Input: part model. Units: mm. Frame: model coordinates. Face numbers are marked on the shaded views. A direction names the side the tool comes from. Give positions to 0.01 mm unless a question says otherwise; leave off trailing zeros. Write each loop counter-clockwise with the first axis right and the second up, starting at its lowest first coordinate (ties: lowest second). Pieces come first, ordered by that corner, then holes. Notation, with made-up numbers: (-27, -11) - (-11, -11) arc R7 cw to (-11, -2) - close; hole circle Ø11 at (-39.75, 84). An arc over 180 degrees is marked (long way). Use a Markdown table: item, result. Add a question column.
1. Set-up query: the marked faces 1 and 2. Return all of +Z, -Z, +X, -X, +Y, -Y with unobstructed straight access to the full face (end or side cutting, diameter ignored); none if empty.
2. Section query A-A, the plane z = -26.67. Return loops of the section in (x, y) (3 decimals).
3. Material intervals for probe 1 along Z at (x, y) = (9.25, 3.25); probe 2 along Z at (x, y) = (7, 2.5); probe 3 along Y at (x, z) = (8.75, -11.43) (3 decimals), sorted ascending.
4. Section query D-D, the plane z = -43.5. Return loops of the section in (x, y), plus the area to 3 significant figures.
5. Pin query (flat end, axial travel): pin 1 (4.5 mm diameter, centred on x = 5.21, z = -33.56, fed in from -Y); pin 2 (1 mm diameter, centred on x = 10, z = -36, fed in from +Y). Return the tip coordinate at first contact, or that it passes through.
6. Section query B-B, the plane x = 18. Count the separate pieces of the cut face and the enclosed holes in it, plus the area to 3 significant figures.
7. Section query C-C, the plane y = 0.5. Return loops of the section in (x, z).
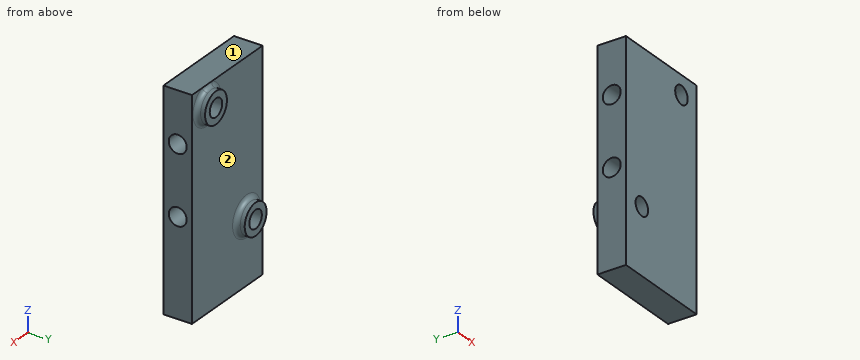
```python
from build123d import *

# Parameters (mm, degrees)
SKETCH1_W           = 22.606
SKETCH1_H           = 48.006
SKETCH1_R           = 2
BOSS_EXTRUDE1_DEPTH = 6.35
SKETCH2_R           = 2
CUT_EXTRUDE1_DEPTH  = 23.606
SKETCH3_R           = 3.5
SKETCH3_R_2         = 2
BOSS_EXTRUDE2_DEPTH = 2
FILLET1_R           = 1


with BuildPart() as part:
    # Sketch1 → Boss-Extrude1 (new body)
    with BuildSketch(Plane(origin=(0, 0, 0), x_dir=(1, 0, 0), z_dir=(0, 1, 0))):
        with Locations((11.43, 24.13)):
            Rectangle(SKETCH1_W, SKETCH1_H)
        with Locations((5.207, 33.55975)):
            Circle(SKETCH1_R, mode=Mode.SUBTRACT)
        with Locations((17.907, 4.34975)):
            Circle(SKETCH1_R, mode=Mode.SUBTRACT)
    extrude(amount=BOSS_EXTRUDE1_DEPTH)

    # Sketch2 → Cut-Extrude1 (cut, through all)
    with BuildSketch(Plane.ZY.offset(-0.127)):
        with Locations((-26.67, 3.175)):
            Circle(SKETCH2_R)
        with Locations((-11.43, 3.175)):
            Circle(SKETCH2_R)
    extrude(amount=-CUT_EXTRUDE1_DEPTH, mode=Mode.SUBTRACT)

    # Sketch3 → Boss-Extrude2 (add)
    with BuildSketch(Plane(origin=(0, 6.35, 0), x_dir=(1, 0, 0), z_dir=(0, 1, 0))):
        with Locations((5.207, 33.55975)):
            Circle(SKETCH3_R)
        with Locations((5.207, 33.55975)):
            Circle(SKETCH3_R_2, mode=Mode.SUBTRACT)
        with Locations((17.907, 4.34975)):
            Circle(SKETCH3_R)
        with Locations((17.907, 4.34975)):
            Circle(SKETCH3_R_2, mode=Mode.SUBTRACT)
    extrude(amount=BOSS_EXTRUDE2_DEPTH)

    # Fillet1
    fillet1_edges = [part.edges().sort_by_distance(p)[0] for p in [
        (1.707, 6.35, -33.55975),
        (14.407, 6.35, -4.34975),
    ]]
    fillet(fillet1_edges, radius=FILLET1_R)


solid = part.part
```
Result sheet:
| question | item | result |
|---|---|---|
| 1 | face 1 | +Z, +X, -X, +Y, -Y |
| 1 | face 2 | +Y |
| 2 | outline | (0.127, 0) - (22.733, 0) - (22.733, 1.175) - (0.127, 1.175) - close; (0.127, 5.175) - (22.733, 5.175) - (22.733, 6.35) - (0.127, 6.35) - close |
| 3 | probe 1 | z = -48.13 to -28.67, -24.67 to -13.43, -9.43 to -0.13 |
| 3 | probe 2 | z = -48.13 to -34.45, -32.67 to -28.55, -24.79 to -13.31, -9.55 to -0.13 |
| 3 | probe 3 | y = 0 to 1.175, 5.175 to 6.35 |
| 4 | outline | (0.13, 0) - (22.73, 0) - (22.73, 6.35) - (0.13, 6.35) - close |
| 4 | area | 144 mm² |
| 5 | pin 1 | stops at y = 0 |
| 5 | pin 2 | stops at y = 6.35 |
| 6 | separate pieces | 2 |
| 6 | enclosed holes | 2 |
| 6 | area | 261 mm² |
| 7 | outline | (0.13, -48.13) - (22.73, -48.13) - (22.73, -0.13) - (0.13, -0.13) - close; hole circle Ø4 at (5.21, -33.56); hole circle Ø4 at (17.91, -4.35) |
